from build123d import *

# Parameters (mm, degrees)
ESQUISSE1_R             = 2.5
BOSS_EXTRU_1_DEPTH      = 10
ENL_V_MAT_EXTRU_1_REACH = 61.034
ESQUISSE2_R             = 2.5
ESQUISSE3_W             = 5
ESQUISSE3_H             = 2.5
ENL_V_MAT_EXTRU_2_DEPTH = 10


with BuildPart() as part:
    # Esquisse1 → Boss.-Extru.1 (new body)
    with BuildSketch(Plane.XY):
        Polygon((-25, -15), (-5, -15), (5, -15), (25, -15), (25, 29.75), (5, 29.75), (5, 15), (-5, 15), (-5, 29.75), (-25, 29.75), align=None)
        with Locations((0, -5)):
            Circle(ESQUISSE1_R, mode=Mode.SUBTRACT)
        with Locations((0, 5)):
            Circle(ESQUISSE1_R, mode=Mode.SUBTRACT)
    extrude(amount=BOSS_EXTRU_1_DEPTH)

    # Enlèv. mat.-Extru.1: up to this face of the body (flat: up to its plane)
    enl_v_mat_extru_1_end = Plane(part.part.faces().sort_by_distance((25, 7.375, 5))[0])
    # Esquisse2 → Enlèv. mat.-Extru.1 (cut, up to the picked face)
    with BuildSketch(Plane.ZY.offset(25), mode=Mode.PRIVATE) as enl_v_mat_extru_1_sk1:
        with Locations((5, 19.75)):
            Circle(ESQUISSE2_R)
    enl_v_mat_extru_1_tool1 = split(extrude(enl_v_mat_extru_1_sk1.sketch, amount=-ENL_V_MAT_EXTRU_1_REACH, mode=Mode.PRIVATE), bisect_by=enl_v_mat_extru_1_end, keep=Keep.BOTH, mode=Mode.PRIVATE)
    # Esquisse2 → Enlèv. mat.-Extru.1 (cut, up to the picked face)
    with BuildSketch(Plane.ZY.offset(25), mode=Mode.PRIVATE) as enl_v_mat_extru_1_sk2:
        Polygon((0, 29.75), (10, 29.75), (10, 23.976497308), align=None)
    enl_v_mat_extru_1_tool2 = split(extrude(enl_v_mat_extru_1_sk2.sketch, amount=-ENL_V_MAT_EXTRU_1_REACH, mode=Mode.PRIVATE), bisect_by=enl_v_mat_extru_1_end, keep=Keep.BOTH, mode=Mode.PRIVATE)
    add(enl_v_mat_extru_1_tool1.solids().sort_by(Axis((-25, 19.75, 5), (1, 0, 0)))[0], mode=Mode.SUBTRACT)
    add(enl_v_mat_extru_1_tool2.solids().sort_by(Axis((-25, 27.825499, 6.666667), (1, 0, 0)))[0], mode=Mode.SUBTRACT)

    # Esquisse3 → Enlèv. mat.-Extru.2 (cut)
    with BuildSketch(Plane.XY.offset(10)):
        with Locations((-15, 9.25)):
            Rectangle(ESQUISSE3_W, ESQUISSE3_H)
        with Locations((-15, -9.25)):
            Rectangle(ESQUISSE3_W, ESQUISSE3_H)
        with Locations((15, -9.25)):
            Rectangle(ESQUISSE3_W, ESQUISSE3_H)
        with Locations((15, 9.25)):
            Rectangle(ESQUISSE3_W, ESQUISSE3_H)
    extrude(amount=-ENL_V_MAT_EXTRU_2_DEPTH, mode=Mode.SUBTRACT)


solid = part.part
Build history of the part. All positions in model axes, mm. A direction names the side the tool comes from. Give positions to 0.01 mm unless a question says otherwise; leave off trailing zeros. Write each loop counter-clockwise with the first axis right and the second up, starting at its lowest first coordinate (ties: lowest second). Pieces come first, ordered by that corner, then holes. Notation, with made-up numbers: (37, 54.25) - (49, 54.25) arc R14 cw to (49, 76.25) - close; hole circle Ø4 at (3, -16.5). An arc over 180 degrees is marked (long way). Use one line per item in the form item = value. Start each with the question number.
1. Two-plate mould, pull along Y, no slides. Class faces 1 (the face through (-17.5, 9, 5)), 2 (the face through (-15, 10.5, 5)), 3 (the face through (-25, 8, 5)), 4 (the face through (-15.14, 26.823, 5.07)): released by +Y, released by -Y, zero draft, split by the parting line, or undercut.
2. Probe line 1 (Y direction, x = 0, z = 5); line 2 (X direction, y = 9, z = 2.75); line 3 (Y direction, x = -17.25, z = 5). List the from-to ranges inside material, lowest first. Write a range as [from, to].
3. Band-saw the part on A-A on x = -14. Write the cut outline in (y, z).
4. Band-saw the part on C-C on z = 4.75. Count the separate pieces of the cut face and the enclosed holes in it, plus the area to 3 significant figures.
5. Band-saw the part on B-B on y = 5. Write the cut outline in (x, z), plus the area to 3 significant figures.
6. Drop flat-ended pins along their axis: pin 1 Ø5 at (x, y) = (-5.5, -3.5) entering from -Z; pin 2 Ø1.5 at (x, z) = (-14, 4) entering from +Y; pin 3 Ø2.5 at (x, z) = (16, 5.5) entering from +Y; pin 4 Ø2.5 at (x, z) = (14, 3.5) entering from +Y. Give the stop position or say it passes through.
7. 3-axis set-ups, long thin cutter, end or side, ignore diameter. For faces 5 (the face through (12.5, 9, 5)), 6 (the face through (5, 22.5, 4.9)), 7 (the face through (14.86, 21.86, 6.34)): which of +Z, -Z, +X, -X, +Y, -Y reach the whole face in a straight line?
8. Band-saw the part on D-D on y = 19.75. Write the cut outline in (x, z).
Conclusion:
q1.face_1 = undercut
q1.face_2 = undercut
q1.face_3 = zero draft
q1.face_4 = released by +Y
q2.line_1 = [-15, -7.5], [-2.5, 2.5], [7.5, 15]
q2.line_2 = [-25, -17.5], [-12.5, 12.5], [17.5, 25]
q2.line_3 = [-15, -10.5], [-8, 8], [10.5, 17.25], [22.25, 26.86]
q3.outline = (-15, 0) - (-10.5, 0) - (-10.5, 10) - (-15, 10) - close; (-8, 0) - (8, 0) - (8, 10) - (-8, 10) - close; (10.5, 0) - (29.75, 0) - (23.98, 10) - (10.5, 10) - close; hole circle Ø5 at (19.75, 5)
q4.separate_pieces = 3
q4.enclosed_holes = 6
q4.area = 1,690 mm²
q5.outline = (-25, 0) - (-2.5, 0) - (-2.5, 10) - (-25, 10) - close; (2.5, 0) - (25, 0) - (25, 10) - (2.5, 10) - close
q5.area = 450 mm²
q6.pin_1 = 0
q6.pin_2 = 27.87
q6.pin_3 = 27.3
q6.pin_4 = 28.45
q7.face_5 = +Z, -Z
q7.face_6 = +Z, -Z, +Y
q7.face_7 = +X, -X
q8.outline = (-25, 0) - (-5, 0) - (-5, 2.5) - (-25, 2.5) - close; (-25, 7.5) - (-5, 7.5) - (-5, 10) - (-25, 10) - close; (5, 0) - (25, 0) - (25, 2.5) - (5, 2.5) - close; (5, 7.5) - (25, 7.5) - (25, 10) - (5, 10) - close
